CAD build for the part. Positions are in the model's coordinates, mm. A direction names the side the tool comes from. Coordinates: 2 decimals unless noted, no trailing zeros. Order: outer loops, then holes, each group sorted by start corner. A loop starts at its lowest first (then second) coordinate and runs counter-clockwise, first axis right, second up. Notation, with made-up numbers: M 43.5,31.25 L 84.5,31.25 A20 ccw 84.5,49.25 Z; hole C -28.75,-9 d2. An arc over 180 degrees is marked long. One line per item, written item: value.
from build123d import *

# Parameters (mm, degrees)
F1_DEPTH = 1100
F3_DEPTH = 125.001
F4_R     = 9
F5_DEPTH = 65.001


with BuildPart() as f1:
    # F0 (on Front) → F1 (new body)
    with BuildSketch(Plane.XZ):
        with BuildLine():
            Line((-25.076735, 63.545803), (-25.076735, -61.454197))
            Line((-25.076735, -61.454197), (39.923265, -61.454197))
            Line((39.923265, -61.454197), (39.923265, -53.954197))
            Line((39.923265, -53.954197), (-12.376735, -53.954197))
            ThreePointArc((-12.376735, -53.954197), (-18.033589, -51.611052), (-20.376735, -45.954197))
            Line((-20.376735, -45.954197), (-20.376735, 48.045803))
            ThreePointArc((-20.376735, 48.045803), (-18.033589, 53.702657), (-12.376735, 56.045803))
            Line((-12.376735, 56.045803), (39.923265, 56.045803))
            Line((39.923265, 56.045803), (39.923265, 63.545803))
            Line((39.923265, 63.545803), (-25.076735, 63.545803))
        make_face()
    extrude(amount=F1_DEPTH)

    # F2 (on face) → F3 (cut, through all)
    with BuildSketch(Plane.XY.offset(63.545803)):
        Polygon((-25.076735, 0), (39.923265, -65), (39.923265, 0), align=None)
        Polygon((-25.076735, -1100), (39.923265, -1100), (39.923265, -1035), align=None)
    extrude(amount=-F3_DEPTH, mode=Mode.SUBTRACT)

    # F4 (on face) → F5 (cut, through all)
    with BuildSketch(Plane(origin=(-25.076735, 0, 0), x_dir=(0, -1, 0), z_dir=(-1, 0, 0))):
        with Locations((32.5, 31.045803)):
            Circle(F4_R)
        with Locations((32.5, -28.954197)):
            Circle(F4_R)
    extrude(amount=-F5_DEPTH, mode=Mode.SUBTRACT)


solid = f1.part
Q1. Slice it at A-A (x = 11). List the corners of the cut face in (y, z), plus the area to 3 significant figures.
Recorded:
outline: M -1063.92,-61.45 L -36.08,-61.45 L -36.08,-53.95 L -1063.92,-53.95 Z; M -1063.92,56.05 L -36.08,56.05 L -36.08,63.55 L -1063.92,63.55 Z
area: 15,400 mm^2
Q2. Slice it at D-D (z = -7). List the corners of the cut face in (x, y), plus the area to 3 significant figures.
Recorded:
outline: M -25.08,-1100 L -20.38,-1095.3 L -20.38,-4.7 L -25.08,0 Z
area: 5,150 mm^2
Q3. Drill centre lines: line 1 along Z through (x, y) = (-21, -32); line 2 along Z through (x, y) = (-21.65, -32.5); line 3 along Z through (x, y) = (27, -469.5). Where is each one in solid material? Low to high.
Recorded:
line 1: z = -61.45 to -37.94, -19.97 to 22.06, 40.03 to 63.55
line 2: z = -61.45 to -37.95, -19.95 to 22.05, 40.05 to 63.55
line 3: z = -61.45 to -53.95, 56.05 to 63.55
Q4. Pin check, flat tips, straight feed: pin 1 Ø16 at (y, z) = (-32.5, 31.05) entering from +X; pin 2 Ø1.5 at (y, z) = (-708, -8.5) entering from +X. Stop position of each tip, or through.
Recorded:
pin 1: passes through
pin 2: stops at x = -20.38
Q5. Which spindle directions (+Z, -Z, +X, -X, +Y, -Y) get a long thin tool onto all of the face, cutting with end or side? Do faces 1 (the face through (14, -542, -53.954)), 2 (the face through (-21.314, -1096.237, -7.922)). Say none if no direction does.
Recorded:
face 1: +X, +Y, -Y
face 2: +Z, -Z, +X, -Y
Q6. Mould opens along Y. For faces 3 (the face through (-22.76, -25.87, 37.13)), 4 (the face through (-22.76, -31.33, -20.03)), 5 (the face through (-21.617, -3.459, 5.967)), 6 (the face through (7, -542, -61.454)) say: released by +Y, released by -Y, zero draft, split by the parting line, or undercut.
Recorded:
face 3: undercut
face 4: undercut
face 5: released by +Y
face 6: zero draft
Q7. Slice it at C-C (y = -853). List the corners of the cut face in (x, z).
Recorded:
outline: M -25.08,-61.45 L 39.92,-61.45 L 39.92,-53.95 L -12.38,-53.95 A8 cw -20.38,-45.95 L -20.38,48.05 A8 cw -12.38,56.05 L 39.92,56.05 L 39.92,63.55 L -25.08,63.55 Z
Q8. Slice it at B-B (y = -32.5). List the corners of the cut face in (x, z), plus the area to 3 significant figures.
Recorded:
outline: M -25.08,-61.45 L 7.42,-61.45 L 7.42,-53.95 L -12.38,-53.95 A8 cw -20.38,-45.95 L -20.38,-37.95 L -25.08,-37.95 Z; M -25.08,-19.95 L -20.38,-19.95 L -20.38,22.05 L -25.08,22.05 Z; M -25.08,40.05 L -20.38,40.05 L -20.38,48.05 A8 cw -12.38,56.05 L 7.42,56.05 L 7.42,63.55 L -25.08,63.55 Z
area: 863 mm^2
